```python
from build123d import *

# Parameters (mm, degrees)
SKETCH1_R                  = 3.175
BOSS_EXTRUDE2_DEPTH        = 3.175
SKETCH2_W                  = 3.175
SKETCH2_H                  = 50.8
BOSS_EXTRUDE3_DEPTH        = 50.8
FILLET3_R                  = 6.35
F_1_2_0_5_DIAMETER_HOLE1_D = 12.7
FILLET4_R                  = 3.175


with BuildPart() as part:
    # Sketch1 → Boss-Extrude2 (new body)
    with BuildSketch(Plane(origin=(0, 0, 0), x_dir=(0, 0, -1), z_dir=(1, 0, 0))):
        with BuildLine():
            Line((0, 0), (-317.5, 0))
            Line((-317.5, 0), (-317.5, 70.920840537))
            ThreePointArc((-317.5, 70.920840537), (-317.227895618, 76.171722787), (-316.414497465, 81.366353538))
            Line((-316.414497465, 81.366353538), (-149.864680249, 874.045513001))
            ThreePointArc((-149.864680249, 874.045513001), (-132.16586597, 903.041552077), (-100.150182785, 914.4))
            Line((-100.150182785, 914.4), (6.35, 914.4))
            Line((6.35, 914.4), (6.35, 863.6))
            Line((6.35, 863.6), (0, 863.6))
            Line((0, 863.6), (0, 101.6))
            Line((0, 101.6), (6.35, 101.6))
            Line((6.35, 101.6), (6.35, 50.8))
            Line((6.35, 50.8), (0, 50.8))
            Line((0, 50.8), (0, 0))
        make_face()
        with Locations((-241.3, 29.604131036)):
            Circle(SKETCH1_R, mode=Mode.SUBTRACT)
        with Locations((-152.4, 29.604131036)):
            Circle(SKETCH1_R, mode=Mode.SUBTRACT)
        with Locations((-158.75, 486.804131036)):
            Circle(SKETCH1_R, mode=Mode.SUBTRACT)
        with Locations((-69.85, 486.804131036)):
            Circle(SKETCH1_R, mode=Mode.SUBTRACT)
    extrude(amount=BOSS_EXTRUDE2_DEPTH)

    # Sketch2 → Boss-Extrude3 (add)
    with BuildSketch(Plane.ZY):
        with Locations((-4.7625, 889)):
            Rectangle(SKETCH2_W, SKETCH2_H)
        with Locations((-4.7625, 76.2)):
            Rectangle(SKETCH2_W, SKETCH2_H)
    extrude(amount=BOSS_EXTRUDE3_DEPTH)

    # Fillet3
    fillet3_edges = [part.edges().sort_by_distance(p)[0] for p in [
        (3.175, 76.2, -6.35),
        (3.175, 889, -6.35),
    ]]
    fillet(fillet3_edges, radius=FILLET3_R)

    # 1_2 _0.5_ Diameter Hole1 (through all)
    with Locations(Plane.XY.offset(-3.175)):
        with Locations((-25.4, 76.2), (-25.4, 889)):
            Hole(F_1_2_0_5_DIAMETER_HOLE1_D / 2)

    # Fillet4
    fillet4_edges = [part.edges().sort_by_distance(p)[0] for p in [
        (0, 889, -3.175),
        (0, 76.2, -3.175),
    ]]
    fillet(fillet4_edges, radius=FILLET4_R)


solid = part.part
```
Geometry check sheet. Reference: the model listing, model coordinates, mm. A direction names the side the tool comes from. Coordinates: 2 decimals unless noted, no trailing zeros. Loops run counter-clockwise (first coordinate to the right, second up) from the corner with the lowest first, then second, coordinate; pieces in that order, holes last. Notation, with made-up numbers: (86.5, -26) - (131.5, -26) arc R14 cw to (131.5, -11) - close; hole circle Ø8 at (5.5, -10.75). An arc over 180 degrees is marked (long way). One line per item, written item: value. Start each with the question number.
(1) Tool access check on faces 1 (the flat face through (3.175, 362, 121)), 2 (the flat face through (-32, 889, -3.175)). Record the directions out of +Z, -Z, +X, -X, +Y, -Y that give a thin tool (end or side, any length) a straight path to the whole face; none if there is none.
(2) Cross-section at B-B on z = 224. Enter the section's corners in (x, y) (3 decimals), plus the area to 3 significant figures.
(3) Depth check by flat-ended pin: P1, Ø3, axis at x = -14, z = -3.5, coming from the -Y side; P2, Ø8, axis at y = 92.5, z = 30.5, coming from the -X side; P3, Ø3.5, axis at x = 1, y = 27, coming from the -Z side. Enter the tip coordinate at first touch or a pass-through.
(4) Cross-section at A-A on y = 548.5. Enter the section's corners in (x, z) (3 decimals), plus the area to 3 significant figures.
(5) Material ranges on line 1 (Y direction, x = -25.4, z = -5.3); line 2 (Y direction, x = 2.3, z = 69.85); line 3 (X direction, y = 663, z = 12) (3 decimals), recorded low to high. Write a range as [from, to].
Results below:
1. face 1: +Z, -Z, +X, +Y, -Y
1. face 2: +Z, -X, +Y, -Y
2. outline: (0, 0) - (3.175, 0) - (3.175, 521.205) - (0, 521.205) - close
2. area: 1,650 mm2
3. P1: stops at y = 50.8
3. P2: stops at x = 0
3. P3: stops at z = 0
4. outline: (0, 0) - (3.175, 0) - (3.175, 218.265) - (0, 218.265) - close
4. area: 693 mm2
5. line 1: y = [50.8, 69.85], [82.55, 101.6], [863.6, 882.65], [895.35, 914.4]
5. line 2: y = [0, 483.63], [489.98, 914.4]
5. line 3: x = [0, 3.175]
